Can you work these out from the drawing? Everything is in mm from the part's minimum corner. Coordinates: 2 decimals unless noted, no trailing zeros. Loops run counter-clockwise (first coordinate to the right, second up) from the corner with the lowest first, then second, coordinate; pieces in that order, holes last. Notation, with made-up numbers: (-39, 13.25) -> (19, 13.25) arc R28 ccw to (19, 44.25) -> close; hole circle Ø11 at (-33, 51.5). An arc over 180 degrees is marked (long way). Put each result on its own line as item: value. Start each with the question number.
Item 1: If we section it at B-B on z = 7.25: Please give me the cut outline in (x, y).
Item 2: Please list where these lines run through material, in increasing order: L1, parallel to X at y = 23, z = 21; L2, parallel to X at y = 15, z = 8.5; L3, parallel to Y at x = 8.5, z = 4. Write a range as from..to.
Item 3: Will these pins go through, and if not, where does the flat tip stop? P1, Ø8, axis at x = 93.5, z = 15.5, coming from the +Y side; P2, Ø1.5, axis at y = 25, z = 2.5, coming from the +X side; P3, Ø6, axis at y = 6.5, z = 14.5, coming from the -X side; P4, Ø1.5, axis at y = 12.5, z = 6, coming from the +X side.
Item 4: If we section it at A-A on y = 32: Please give me the cut outline in (x, z), plus the area to 3 significant figures.
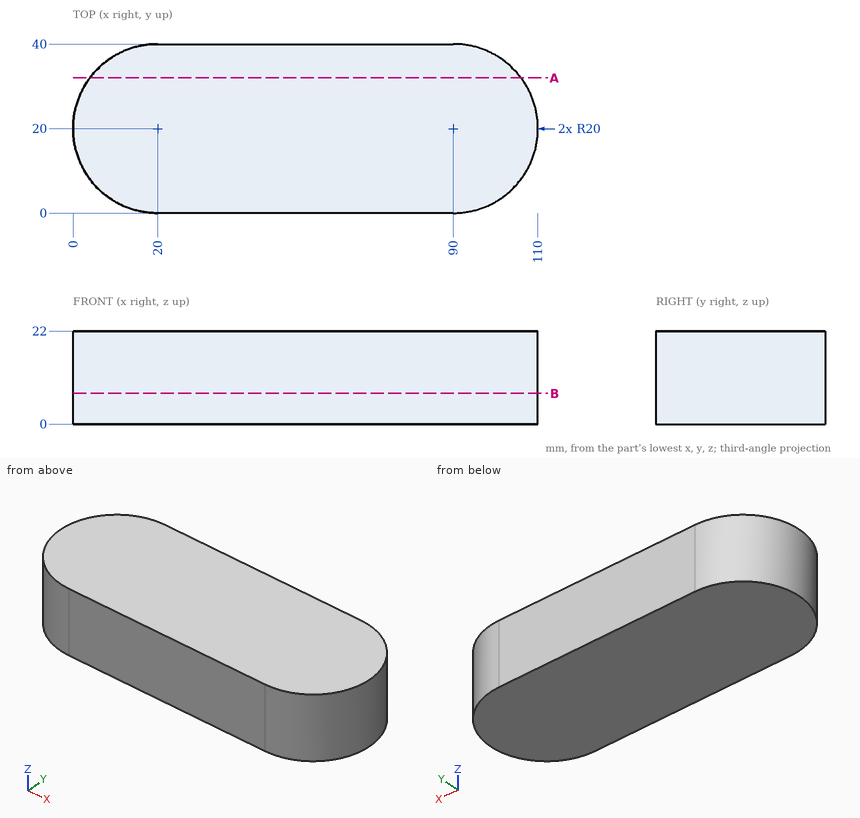
Solutions:
1. outline: (20, 0) -> (90, 0) arc R20 ccw to (90, 40) -> (20, 40) arc R20 ccw to start
2. L1: 0.23..109.77
2. L2: 0.64..109.36
2. L3: 3.64..36.36
3. P1: y = 40
3. P2: x = 109.54
3. P3: x = 2.98
3. P4: x = 108.83
4. outline: (4, 0) -> (106, 0) -> (106, 22) -> (4, 22) -> close
4. area: 2,240 mm^2
